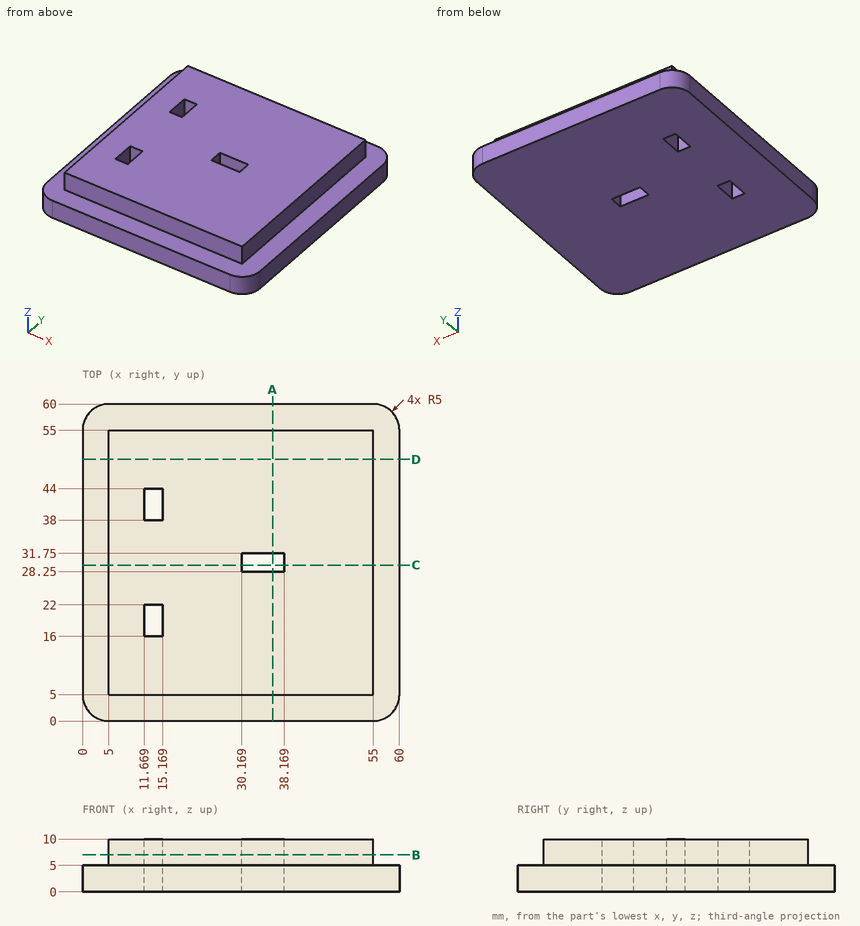
Here's the drawing with two shaded views (mm, measured from the low corner). I have some questions. Give positions to 0.01 mm unless a question says otherwise; leave off trailing zeros. Loops run counter-clockwise (first coordinate to the right, second up) from the corner with the lowest first, then second, coordinate; pieces in that order, holes last. Notation, with made-up numbers: M -22,32.25 L -5,32.25 A13 cw -5,37.25 Z; hole C 17,39.25 d8. An arc over 180 degrees is marked long. One line per item, written item: value.
1) Imagine slicing it at D-D on y = 49.5. Write out the boundary of the cut face in (x, z).
Geometry check:
outline: M 0,0 L 60,0 L 60,5 L 55,5 L 55,10 L 5,10 L 5,5 L 0,5 Z
2) Imagine slicing it at B-B on z = 7. Write out the boundary of the cut face in (x, y).
Geometry check:
outline: M 5,5 L 55,5 L 55,55 L 5,55 Z; hole M 11.67,16 L 15.17,16 L 15.17,22 L 11.67,22 Z; hole M 11.67,38 L 15.17,38 L 15.17,44 L 11.67,44 Z; hole M 30.17,28.25 L 38.17,28.25 L 38.17,31.75 L 30.17,31.75 Z
3) Imagine slicing it at C-C on y = 29.5. Write out the boundary of the cut face in (x, z), and give its area (3 significant figures).
Geometry check:
outline: M 0,0 L 30.17,0 L 30.17,10 L 5,10 L 5,5 L 0,5 Z; M 38.17,0 L 60,0 L 60,5 L 55,5 L 55,10 L 38.17,10 Z
area: 470 mm²
4) Imagine slicing it at A-A on x = 36. Write out the boundary of the cut face in (y, z).
Geometry check:
outline: M 0,0 L 28.25,0 L 28.25,10 L 5,10 L 5,5 L 0,5 Z; M 31.75,0 L 60,0 L 60,5 L 55,5 L 55,10 L 31.75,10 Z
5) Please list where these lines run through material, in increasing order: line 1 (Y direction, x = 43, z = 8.75); line 2 (X direction, y = 42.5, z = 6.75); line 3 (Z direction, x = 56.5, y = 18).
Geometry check:
line 1: y = 5 to 55
line 2: x = 5 to 11.67, 15.17 to 55
line 3: z = 0 to 5
6) I'm going to push flat-ended pins straight in: pin 1 (5.5 mm diameter, centred on y = 29.5, z = 7.5, fed in from -X); pin 2 (5.5 mm diameter, centred on x = 42, z = 8, fed in from -Y); pin 3 (5.5 mm diameter, centred on y = 32, z = 8, fed in from +X). Where does each tip first touch, or does it pass through?
Geometry check:
pin 1: stops at x = 0
pin 2: stops at y = 5
pin 3: stops at x = 55
